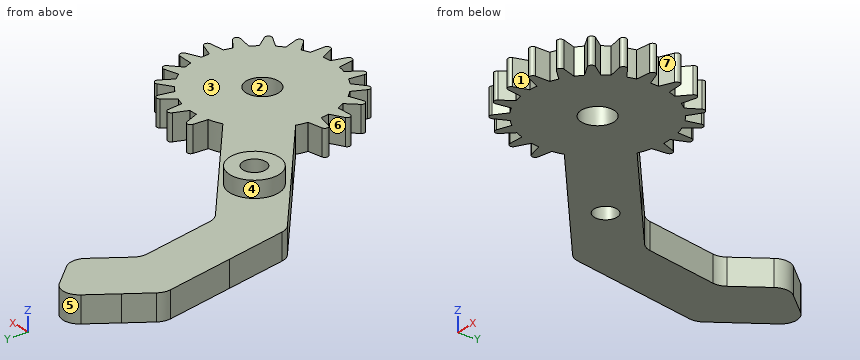
Autodesk Inventor part; units mm, degrees
ref_plane "YZ Plane" through (0, 0, 0) normal (1, 0, 0) x (0, 1, 0)
ref_plane "XZ Plane" through (0, 0, 0) normal (0, 1, 0) x (-1, 0, 0)
ref_plane "XY Plane" through (0, 0, 0) normal (0, 0, 1) x (1, 0, 0)
sketch "Sketch1" plane through (0, 0, 0) normal (0, 0, 1) x (1, 0, 0)
  circle A0 centre (0, 0) radius 2.5
  line L0 (0, 0) -> (-15.5714, 12.5511)
  line L1 (0, 0) -> (20, 0) construction
  line L2 (-15.5714, 12.5511) -> (-18.3421, 9.1137)
  line L3 (0, 0) -> (-10.3273, 2.6535)
  line L4 (0, 0) -> (26.0413, 0) construction
  line L5 (-18.3421, 9.1137) -> (-10.3273, 2.6535)
  line L6 (-23.1447, 24.3261) -> (-21.5758, 26.2725)
  circle A1 centre (-21.5758, 26.2725) radius 2.5
  line L7 (-23.6708, 23.9703) -> (-17.7415, 23.9703) construction
  line L8 (-24.0288, 25.7899) -> (-26.2178, 36.9166)
  line L9 (-24.0288, 25.7899) -> (-12.6888, 25.7899) construction
  line L10 (-26.2178, 36.9166) -> (-23.7649, 37.3992)
  circle A2 centre (-23.7649, 37.3992) radius 2.5
  line L11 (-26.2069, 38.2378) -> (-20.9991, 38.2378) construction
  line L12 (-25.8513, 38.7765) -> (-22.6835, 43.5752)
  line L13 (-25.8513, 38.7765) -> (-20.1013, 38.7765) construction
  line L14 (-22.6835, 43.5752) -> (-24.7699, 44.9525)
  circle A3 centre (-24.7699, 44.9525) radius 2.5
  line L15 (0, 0) -> (60, 0) construction
  line L16 (-25.9313, 49.9817) -> (-22.9112, 46.6245)
  line L17 (-24.7699, 40.4146) -> (-32.5897, 45.5767)
  line L18 (-32.5897, 45.5767) -> (-29.8763, 49.6871)
  line L19 (-32.5897, 45.5767) -> (-34.946, 42.0073)
  line L20 (-25.1233, 31.3533) -> (-33.2672, 29.7511)
  line L21 (-33.2672, 29.7511) -> (-35.3126, 40.1474)
  line L22 (-33.2672, 29.7511) -> (-31.4304, 20.4146)
  line L23 (-18.3421, 9.1137) -> (-30.5463, 18.9507)
  line L24 (-16.7222, 19.1493) -> (-22.2635, 12.2745)
  arc A4 (-10.3273, 2.6535) -> (-4.786, 9.5283) centre (0, 0) ccw
  arc A5 (-25.9313, 49.9817) -> (-29.8763, 49.6871) centre (-27.7899, 48.3098) ccw
  arc A6 (-34.946, 42.0073) -> (-35.3126, 40.1474) centre (-32.8596, 40.63) ccw
  arc A7 (-31.4304, 20.4146) -> (-30.5463, 18.9507) centre (-28.9774, 20.8971) ccw
  line L25 (-16.7222, 19.1493) -> (-23.1447, 24.3261)
  line L26 (-16.7222, 19.1493) -> (-4.786, 9.5283)
  circle A8 centre (-19.4928, 15.7119) radius 1.75
  line L27 (0, 0) -> (-10.6628, 0)
  line L28 (-4.786, 9.5283) -> (0, 0)
  arc A9 (-12.7774, 0.4964) -> (-12.7774, -0.4964) centre (-12.6628, 0) ccw
  line L29 (-10.6628, 0) -> (-10.1628, 0)
  line L30 (-10.6162, 0.9953) -> (-12.7774, 0.4964)
  line L31 (-10.6162, -0.9953) -> (-12.7774, -0.4964)
  line L32 (-10.4242, -2.2431) -> (-12.3353, -3.3688)
  line L33 (-9.8256, -4.1416) -> (-12.0367, -4.3157)
  arc A10 (-12.3353, -3.3688) -> (-12.0367, -4.3157) centre (-12.0767, -3.8078) ccw
  line L34 (-9.2672, -5.2739) -> (-10.7513, -6.9222)
  line L35 (-8.1254, -6.9045) -> (-10.1819, -7.7354)
  arc A11 (-10.7513, -6.9222) -> (-10.1819, -7.7354) centre (-10.3727, -7.2631) ccw
  line L36 (-7.2524, -7.8165) -> (-8.1722, -9.8348)
  line L37 (-5.6731, -9.0283) -> (-7.3845, -10.4392)
  arc A12 (-8.1722, -9.8348) -> (-7.3845, -10.4392) centre (-7.7086, -10.046) ccw
  line L38 (-4.5663, -9.6356) -> (-4.8366, -11.837)
  line L39 (-2.6957, -10.3164) -> (-3.9036, -12.1766)
  arc A13 (-4.8366, -11.837) -> (-3.9036, -12.1766) centre (-4.3309, -11.8991) ccw
  line L40 (-1.4574, -10.5627) -> (-1.0533, -12.7435)
  line L41 (0.5313, -10.6495) -> (-0.0614, -12.7869)
  arc A14 (-1.0533, -12.7435) -> (-0.0614, -12.7869) centre (-0.5523, -12.6507) ccw
  line L42 (1.7863, -10.5121) -> (2.8275, -12.4705)
  line L43 (3.7091, -9.9969) -> (3.7865, -12.2135)
  arc A15 (2.8275, -12.4705) -> (3.7865, -12.2135) centre (3.2774, -12.2313) ccw
  line L44 (4.8646, -9.4884) -> (6.4466, -11.043)
  line L45 (6.5435, -8.4188) -> (7.2839, -10.5096)
  arc A16 (6.4466, -11.043) -> (7.2839, -10.5096) centre (6.8037, -10.6797) ccw
  line L46 (7.4927, -7.5864) -> (9.4689, -8.5934)
  line L47 (8.7723, -6.0615) -> (10.1071, -7.8329)
  arc A17 (9.4689, -8.5934) -> (10.1071, -7.8329) centre (9.7002, -8.1395) ccw
  line L48 (9.4272, -4.9822) -> (11.6148, -5.3483)
  line L49 (10.189, -3.1431) -> (11.9947, -4.4311)
  arc A18 (11.6148, -5.3483) -> (11.9947, -4.4311) centre (11.6989, -4.8458) ccw
  line L50 (10.4891, -1.9168) -> (12.6855, -1.6081)
  line L51 (10.6626, 0.0663) -> (12.772, -0.6191)
  arc A19 (12.6855, -1.6081) -> (12.772, -0.6191) centre (12.6146, -1.1036) ccw
  line L52 (10.58, 1.326) -> (12.5819, 2.2809)
  line L53 (10.1491, 3.2695) -> (12.367, 3.2502)
  arc A20 (12.5819, 2.2809) -> (12.367, 3.2502) centre (12.3626, 2.7407) ccw
  line L54 (9.6916, 4.4461) -> (11.3137, 5.9588)
  line L55 (8.6962, 6.1701) -> (10.8173, 6.8186)
  arc A21 (11.3137, 5.9588) -> (10.8173, 6.8186) centre (10.9663, 6.3314) ccw
  line L56 (7.906, 7.1547) -> (8.9982, 9.0851)
  line L57 (6.4384, 8.4995) -> (8.2663, 9.7558)
  arc A22 (8.9982, 9.0851) -> (8.2663, 9.7558) centre (8.5548, 9.336) ccw
  line L58 (5.3887, 9.2009) -> (5.8498, 11.3704)
  line L59 (3.5845, 10.0422) -> (4.9501, 11.79)
  arc A23 (5.8498, 11.3704) -> (4.9501, 11.79) centre (5.3515, 11.4764) ccw
  line L60 (2.3725, 10.3955) -> (2.1599, 12.6033)
  line L61 (0.3989, 10.6553) -> (1.1756, 12.7328)
  arc A24 (2.1599, 12.6033) -> (1.1756, 12.7328) centre (1.6528, 12.5544) ccw
  line L62 (-0.8633, 10.6278) -> (-1.7299, 12.6694)
  line L63 (-2.8237, 10.2821) -> (-2.7076, 12.497)
  arc A25 (-1.7299, 12.6694) -> (-2.7076, 12.497) centre (-2.1989, 12.4704) ccw
  point P0 (-10.1693, -3.2064)
  point P1 (-8.7344, -6.1159)
  point P2 (-6.4911, -8.4593)
  point P3 (-3.6469, -10.0197)
  point P4 (-0.4651, -10.6526)
  point P5 (2.7597, -10.2994)
  point P6 (5.7291, -8.9929)
  point P7 (8.1681, -6.8539)
  point P8 (9.8511, -4.0805)
  point P9 (10.6222, -0.9293)
  point P10 (10.41, 2.3078)
  point P11 (9.2342, 5.3314)
  point P12 (7.2037, 7.8614)
  point P13 (4.5063, 9.6637)
  point P14 (1.3918, 10.5715)
  point P15 (-1.8516, 10.5008)
  dimension "d0" = 5
  dimension "d1" = 20
  dimension "d2" = 141.13
  dimension "d3" = 4.415
  dimension "d4" = 165.59
  dimension "d6" = 10.2942
  dimension "d8" = 2.5
  dimension "d11" = 11.34
  dimension "d13" = 101.13
  dimension "d14" = 2.5
  dimension "d16" = 5.75
  dimension "d17" = 56.57
  dimension "d18" = 2.5
  dimension "d22" = 9.37
  dimension "d23" = 8.3
  dimension "d25" = 8.83
  dimension "d26" = 2.5
  dimension "d27" = 3.5
  dimension "d34" = 63.33
  dimension "d41" = 0.5
  dimension "d46" = 280
extrude "Extrusion1" add sketch "Sketch1" along normal blind 4 contours A0 L28 A4 L27 | A0 L0 L2 L23 L24 A8 L26 L28 | L27 A4 L3 A0 | A0 L3 L5 L2 L0 | L63 A25 L62 A4 | L24 A8 L23 A7 L22 L20 L8 A1 L25 | A4 L31 A9 L30 | L61 A24 L60 A4 | A4 L33 A10 L32 | L20 L21 A6 L19 L17 L12 A2 L8 | L59 A23 L58 A4 | A4 L35 A11 L34 | L57 A22 L56 A4 | L17 L18 A5 L16 A3 L12 | A4 L37 A12 L36 | A3 | L55 A21 L54 A4 | A4 L39 A13 L38 | L53 A20 L52 A4 | A4 L41 A14 L40 | L51 A19 L50 A4 | A4 L43 A15 L42 | L49 A18 L48 A4 | A4 L45 A16 L44 | L47 A17 L46 A4
sketch "Sketch2" plane through (0, 0, 4) normal (0, 0, 1) x (1, 0, 0)
  circle A0 centre (-19.4928, 15.7119) radius 1.75
  circle A1 centre (-19.4928, 15.7119) radius 1.75
  circle A2 centre (-19.4928, 15.7119) radius 3.75
  point P0 (0, 0)
  dimension "d50" = 7.5
extrude "Extrusion2" add sketch "Sketch2" along normal blind 2.5
sketch "Sketch3" plane through (0, 0, 4) normal (0, 0, 1) x (1, 0, 0)
  circle A0 centre (0, 0) radius 2.5
  arc A1 (3.5845, 10.0422) -> (2.3725, 10.3955) centre (0, 0) ccw
  arc A2 (6.4384, 8.4995) -> (5.3887, 9.2009) centre (0, 0) ccw
  line L0 (3.5845, 10.0422) -> (5.3887, 9.2009)
  arc A3 (5.8498, 11.3704) -> (4.9501, 11.79) centre (5.3515, 11.4764) ccw
  line L1 (4.4866, 9.6215) -> (5.3515, 11.4764)
  dimension "d53" = 1.9906
  dimension "d54" = 2.0466
properties part number "Servo pinza 2"
The model under review builds one solid part; all positions refer to its coordinate system, in mm. Face numbers are marked on the shaded views. A direction names the side the tool comes from. Coordinates: 2 decimals unless noted, no trailing zeros. Loops run counter-clockwise (first coordinate to the right, second up) from the corner with the lowest first, then second, coordinate; pieces in that order, holes last.
(1) Wall thickness on L1, parallel to X at y = 15, z = 6; L2, parallel to X at y = 2, z = 1; L3, parallel to Y at x = -1, z = 1.5: over which ranges is each line inside the solid? List them lowest first.
Determined:
L1: x = -23.17 to -21.09, -17.89 to -15.81
L2: x = -10.47 to -1.5, 1.5 to 11.99
L3: y = -12.89 to -2.29, 2.29 to 10.95
(2) Consider section B-B, the plane y = 15. Give the boundary of the cut face in (x, z).
Determined:
outline: (-25.64, 0) - (-21.09, 0) - (-21.09, 6.5) - (-23.17, 6.5) - (-23.17, 4) - (-25.64, 4) - close; (-17.89, 0) - (-11.57, 0) - (-11.57, 4) - (-15.81, 4) - (-15.81, 6.5) - (-17.89, 6.5) - close
(3) Consider section A-A, the plane x = -20. Give the boundary of the cut face in (y, z), plus the area to 3 significant figures.
Determined:
outline: (10.45, 0) - (14.04, 0) - (14.04, 6.5) - (12, 6.5) - (12, 4) - (10.45, 4) - close; (17.39, 0) - (21.79, 0) - (21.79, 4) - (19.43, 4) - (19.43, 6.5) - (17.39, 6.5) - close
area: 42.2 mm2
(4) Tool access review of the marked faces 5, 6 and 7: name each direction out of +Z, -Z, +X, -X, +Y, -Y from which nothing blocks a thin tool from reaching the whole face with its end or side.
Determined:
face 5: +Z, -Z, +Y
face 6: +Z, -Z, -X
face 7: +Z, -Z, +X
(5) Consider section C-C, the plane z = 3.25. Give the number of separate pieces and of enclosed holes in the cut face, plus the area to 3 significant figures.
Determined:
separate pieces: 1
enclosed holes: 2
area: 855 mm2
(6) Draft analysis for pull direction X (two halves, no side actions). For the marked faces 1, 2, 3 and 4, state which applies: +X half, -X half, draft (parallel to the pull), parting line (faces both ways), or undercut.
Determined:
face 1: undercut
face 2: undercut
face 3: draft
face 4: parting line
(7) Insertion check: P1, Ø1.5, axis at y = 36.5, z = 2, coming from the +X side; P2, Ø1.5, axis at x = -22, y = 26.5, coming from the -Z side; P3, Ø1, axis at x = -14, z = 2, coming from the +Y side; P4, Ø3, axis at x = -4.5, z = 3.5, coming from the +Y side. Each pin has a flat end and moves straight along its axis. Give the tip position at first contact, or say it passes through.
Determined:
P1: stops at x = -25.99
P2: passes through
P3: stops at y = 17.36
P4: stops at y = 10.51
